Design review of the part built by this model. Coordinates are the model's own, in mm. A direction names the side the tool comes from. Coordinates: 2 decimals unless noted, no trailing zeros. Loops run counter-clockwise (first coordinate to the right, second up) from the corner with the lowest first, then second, coordinate; pieces in that order, holes last. Notation, with made-up numbers: (27, -34.5) - (84, -34.5) arc R21 cw to (84, -13.5) - close; hole circle Ø3 at (76.25, 38). An arc over 180 degrees is marked (long way). One line per question, with ' | ' between items.
from build123d import *

# Parameters (mm, degrees)
F1_DEPTH = 30
F1_TAPER = 3
F2_DEPTH = 30
F3_START = 20
F3_DEPTH = 10


with BuildPart() as f1:
    # F0 (on Top) → F1 (new body)
    with BuildSketch(Plane.XY):
        with BuildLine():
            Line((265.848302468, 214.8965468303), (85.848302468, 214.8965468303))
            Line((85.848302468, 214.8965468303), (85.848302468, 114.8965468303))
            Line((85.848302468, 114.8965468303), (285.848302468, 114.8965468303))
            Line((285.848302468, 114.8965468303), (285.848302468, 194.8965468303))
            ThreePointArc((285.848302468, 194.8965468303), (279.9904380917, 209.0386824541), (265.848302468, 214.8965468303))
        make_face()
        with BuildLine():
            Line((260.6931902693, 154.8965468303), (111.0034146666, 154.8965468303))
            ThreePointArc((111.0034146666, 154.8965468303), (101.0034146666, 164.8965468303), (111.0034146666, 174.8965468303))
            Line((111.0034146666, 174.8965468303), (260.6931902693, 174.8965468303))
            ThreePointArc((260.6931902693, 174.8965468303), (270.6931902693, 164.8965468303), (260.6931902693, 154.8965468303))
        make_face(mode=Mode.SUBTRACT)
        with BuildLine():
            ThreePointArc((111.0034146666, 174.8965468303), (101.0034146666, 164.8965468303), (111.0034146666, 154.8965468303))
            Line((111.0034146666, 154.8965468303), (260.6931902693, 154.8965468303))
            ThreePointArc((260.6931902693, 154.8965468303), (270.6931902693, 164.8965468303), (260.6931902693, 174.8965468303))
            Line((260.6931902693, 174.8965468303), (111.0034146666, 174.8965468303))
        make_face()
        with BuildLine():
            Line((260.6931902693, 159.8965468303), (111.0034146666, 159.8965468303))
            ThreePointArc((111.0034146666, 159.8965468303), (106.0034146666, 164.8965468303), (111.0034146666, 169.8965468303))
            Line((111.0034146666, 169.8965468303), (260.6931902693, 169.8965468303))
            ThreePointArc((260.6931902693, 169.8965468303), (265.6931902693, 164.8965468303), (260.6931902693, 159.8965468303))
        make_face(mode=Mode.SUBTRACT)
        with BuildLine():
            ThreePointArc((111.0034146666, 169.8965468303), (106.0034146666, 164.8965468303), (111.0034146666, 159.8965468303))
            Line((111.0034146666, 159.8965468303), (260.6931902693, 159.8965468303))
            ThreePointArc((260.6931902693, 159.8965468303), (265.6931902693, 164.8965468303), (260.6931902693, 169.8965468303))
            Line((260.6931902693, 169.8965468303), (111.0034146666, 169.8965468303))
        make_face()
    extrude(amount=F1_DEPTH, taper=F1_TAPER)

    # F0 (on Top) → F2 (cut)
    with BuildSketch(Plane.XY):
        with BuildLine():
            ThreePointArc((111.0034146666, 169.8965468303), (106.0034146666, 164.8965468303), (111.0034146666, 159.8965468303))
            Line((111.0034146666, 159.8965468303), (260.6931902693, 159.8965468303))
            ThreePointArc((260.6931902693, 159.8965468303), (265.6931902693, 164.8965468303), (260.6931902693, 169.8965468303))
            Line((260.6931902693, 169.8965468303), (111.0034146666, 169.8965468303))
        make_face()
    extrude(amount=F2_DEPTH, mode=Mode.SUBTRACT)

    # F0 (on Top) → F3 (cut)
    with BuildSketch(Plane.XY.offset(F3_START)):
        with BuildLine():
            ThreePointArc((111.0034146666, 174.8965468303), (101.0034146666, 164.8965468303), (111.0034146666, 154.8965468303))
            Line((111.0034146666, 154.8965468303), (260.6931902693, 154.8965468303))
            ThreePointArc((260.6931902693, 154.8965468303), (270.6931902693, 164.8965468303), (260.6931902693, 174.8965468303))
            Line((260.6931902693, 174.8965468303), (111.0034146666, 174.8965468303))
        make_face()
        with BuildLine():
            Line((260.6931902693, 159.8965468303), (111.0034146666, 159.8965468303))
            ThreePointArc((111.0034146666, 159.8965468303), (106.0034146666, 164.8965468303), (111.0034146666, 169.8965468303))
            Line((111.0034146666, 169.8965468303), (260.6931902693, 169.8965468303))
            ThreePointArc((260.6931902693, 169.8965468303), (265.6931902693, 164.8965468303), (260.6931902693, 159.8965468303))
        make_face(mode=Mode.SUBTRACT)
    extrude(amount=F3_DEPTH, mode=Mode.SUBTRACT)


solid = f1.part
Q1. For pin 1 (10 mm diameter, centred on x = 193, z = 24.5, fed in from +Y); pin 2 (8 mm diameter, centred on x = 207, z = 23.5, fed in from -Y); pin 3 (1.5 mm diameter, centred on y = 148, z = 25.5, fed in from -X), all flat-tipped, find the tip position at first contact; note any pin that passes through.
Returned:
pin 1: stops at y = 213.87 | pin 2: stops at y = 115.92 | pin 3: stops at x = 87.15
Q2. Draft analysis for pull direction X (two halves, no side actions). For faces 4 (the flat face through (184, 176, 30)), 5 (the flat face through (285.073, 155.457, 14.79)), 6 (the flat face through (86.623, 164.197, 14.79)), 7 (the cylindrical face through (265.692, 164.787, 9.86)), state which applies: +X half, -X half, draft (parallel to the pull), parting line (faces both ways), or undercut.
Returned:
face 4: draft | face 5: +X half | face 6: -X half | face 7: undercut
Q3. Take a section at B-B (z = 7). Give the boundary of the cut face in (x, y).
Returned:
outline: (86.22, 115.26) - (285.48, 115.26) - (285.48, 194.9) arc R19.63 ccw to (265.85, 214.53) - (86.22, 214.53) - close; hole (111, 159.9) - (260.69, 159.9) arc R5 ccw to (260.69, 169.9) - (111, 169.9) arc R5 ccw to start
Q4. To check wall thickness, follow line 1 along Y through (x, z) = (176.5, 18); line 2 along X through (y, z) = (170.5, 24); line 3 along Y through (x, z) = (107, 18.5). State the ranges of each line that lie inside material, in increasing order.
Returned:
line 1: y = 115.84 to 159.9, 169.9 to 213.95 | line 2: x = 87.11 to 102.72, 268.98 to 284.59 | line 3: y = 115.87 to 161.9, 167.89 to 213.93
Q5. Take a section at C-C (z = 23.5). Give the boundary of the cut face in (x, y), plus the area to 3 significant figures.
Returned:
outline: (87.08, 116.13) - (284.62, 116.13) - (284.62, 194.9) arc R18.77 ccw to (265.85, 213.66) - (87.08, 213.66) - close; hole (111, 154.9) - (260.69, 154.9) arc R10 ccw to (260.69, 174.9) - (111, 174.9) arc R10 ccw to start | area: 15,900 mm²
Q6. Tool access review of faces 1 (the cylindrical face through (101.006, 165.116, 24.93)), 2 (the flat face through (184, 154, 0)), 3 (the flat face through (185, 159.897, 10)): name each direction out of +Z, -Z, +X, -X, +Y, -Y from which nothing blocks a thin tool from reaching the whole face with its end or side.
Returned:
face 1: +Z | face 2: -Z, +X, -X, +Y, -Y | face 3: +Z, -Z
Q7. Take a section at A-A (x = 137). Give the boundary of the cut face in (y, z).
Returned:
outline: (114.9, 0) - (159.9, 0) - (159.9, 20) - (154.9, 20) - (154.9, 30) - (116.47, 30) - close; (169.9, 0) - (214.9, 0) - (213.32, 30) - (174.9, 30) - (174.9, 20) - (169.9, 20) - close
